```python
from build123d import *

# Parameters (mm, degrees)
SKETCH1_R                       = 33.5
SKETCH1_R_2                     = 17
BOSS_EXTRUDE1_DEPTH             = 6
F_4_0MM_DOWEL_HOLE1_D           = 4
F_4_0MM_DOWEL_HOLE1_DEPTH       = 24.5
F_4_0MM_DOWEL_HOLE1_CSINK_D     = 4.05
F_4_0MM_DOWEL_HOLE1_CSINK_ANGLE = 90
F_4_0MM_DOWEL_HOLE1_TIP         = 1.201721238


with BuildPart() as part:
    # Sketch1 → Boss-Extrude1 (new body)
    with BuildSketch(Plane.XY):
        Circle(SKETCH1_R)
        Circle(SKETCH1_R_2, mode=Mode.SUBTRACT)
    extrude(amount=BOSS_EXTRUDE1_DEPTH)

    # Ø4.0mm Dowel Hole1
    with Locations(Plane(origin=(28.5, 0, 0), x_dir=(-1, 0, 0), z_dir=(0, 0, -1))):
        with Locations((0, 0), (14.25, 24.681724008), (42.75, 24.681724008), (57, 0), (42.75, -24.681724008), (14.25, -24.681724008)):
            CounterSinkHole(F_4_0MM_DOWEL_HOLE1_D / 2, F_4_0MM_DOWEL_HOLE1_CSINK_D / 2, depth=F_4_0MM_DOWEL_HOLE1_DEPTH, counter_sink_angle=F_4_0MM_DOWEL_HOLE1_CSINK_ANGLE)
            with Locations((0, 0, -(F_4_0MM_DOWEL_HOLE1_DEPTH + F_4_0MM_DOWEL_HOLE1_TIP / 2))):  # 118° drill point
                Cone(0, F_4_0MM_DOWEL_HOLE1_D / 2, F_4_0MM_DOWEL_HOLE1_TIP, mode=Mode.SUBTRACT)


solid = part.part
```
Geometry: final body of the model. Coordinates: model frame, mm. Round coordinates to 2 decimals unless told otherwise and drop trailing zeros. Order: outer loops, then holes, each group sorted by start corner. A loop starts at its lowest first (then second) coordinate and runs counter-clockwise, first axis right, second up. Notation, with made-up numbers: (17.25, 79.5) - (49.25, 79.5) arc R19 cw to (49.25, 91.5) - close; hole circle Ø7 at (46.5, -36.5). An arc over 180 degrees is marked (long way). Use CSV: the item, a comma, the result in double quotes. Start each with the question number.
Q1. Material intervals for line 1 along Y through (x, z) = (-14.25, 4.1); line 2 along X through (y, z) = (-26, 4.9); line 3 along Y through (x, z) = (-14, 3.3), sorted ascending. Write a range as from..to.
Q2. Section query A-A (y = 0). Return loops of the section in (x, z) (3 decimals), and give its area (3 significant figures).
Q3. Section query D-D (x = 14.25). Return loops of the section in (y, z) (3 decimals), and give its area (3 significant figures).
Q4. Mould query, pull axis Y, two halves, no side actions, for faces 1 (the face through (-15.4, 7.9, 6)), 2 (the face through (-7.262, -32.703, 2.958)), 3 (the face through (30.408, 0.601, 3.054)). Classes: +Y half, -Y half, draft (parallel to the pull), parting line (faces both ways), or undercut.
Q5. Section query B-B (x = 0). Return loops of the section in (y, z), and give its area (3 significant figures).
Q6. Section query C-C (z = 4.65). Return loops of the section in (x, y).
Q7. First-contact query: pin 1 (3 mm diameter, centred on x = 22, z = 1, fed in from -Y); pin 2 (1.5 mm diameter, centred on x = -26.5, z = 5, fed in from -Y). Flat tips, straight axial feed; report the tip coordinate or a pass-through.
Result set:
1,line 1,"y = -30.32..-26.68, -22.68..-9.27, 9.27..22.68, 26.68..30.32"
1,line 2,"x = -21.12..-15.75, -12.75..12.75, 15.75..21.12"
1,line 3,"y = -30.43..-26.67, -22.7..-9.64, 9.64..22.7, 26.67..30.43"
2,outline,"(-33.5, 0) - (-30.525, 0) - (-30.5, 0.025) - (-30.5, 6) - (-33.5, 6) - close; (-26.5, 0.025) - (-26.475, 0) - (-17, 0) - (-17, 6) - (-26.5, 6) - close; (17, 0) - (26.475, 0) - (26.5, 0.025) - (26.5, 6) - (17, 6) - close; (30.5, 0.025) - (30.525, 0) - (33.5, 0) - (33.5, 6) - (30.5, 6) - close"
2,area,"150 mm2"
3,outline,"(-30.318, 0) - (-26.707, 0) - (-26.682, 0.025) - (-26.682, 6) - (-30.318, 6) - close; (-22.682, 0.025) - (-22.657, 0) - (-9.27, 0) - (-9.27, 6) - (-22.682, 6) - close; (9.27, 0) - (22.657, 0) - (22.682, 0.025) - (22.682, 6) - (9.27, 6) - close; (26.682, 0.025) - (26.707, 0) - (30.318, 0) - (30.318, 6) - (26.682, 6) - close"
3,area,"205 mm2"
4,face 1,"draft"
4,face 2,"parting line"
4,face 3,"undercut"
5,outline,"(-33.5, 0) - (-17, 0) - (-17, 6) - (-33.5, 6) - close; (17, 0) - (33.5, 0) - (33.5, 6) - (17, 6) - close"
5,area,"198 mm2"
6,outline,"circle Ø67 at (0, 0); hole circle Ø4 at (-28.5, 0); hole circle Ø34 at (0, 0); hole circle Ø4 at (-14.25, -24.68); hole circle Ø4 at (-14.25, 24.68); hole circle Ø4 at (14.25, -24.68); hole circle Ø4 at (14.25, 24.68); hole circle Ø4 at (28.5, 0)"
7,pin 1,"stops at y = -26.5"
7,pin 2,"stops at y = -21.43"
